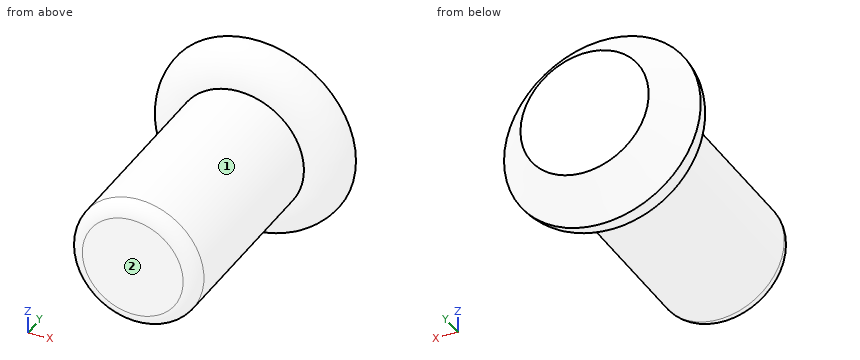
from build123d import *

# Parameters (mm, degrees)
F1_R     = 36.4721508719
F2_DEPTH = 25.399999693
F3_SIZE  = 12.7
F4_R     = 12.69999
F5_R     = 23.7721508719
F6_DEPTH = 101.6
F7_R     = 5.08


# Not quite as in the source:
# - a fillet or chamfer is up to 0.001 mm smaller than in the source, because OpenCascade refuses the exact size


with BuildPart() as f2:
    # F1 (on face) → F2 (new body)
    with BuildSketch(Plane.XZ):
        with Locations((27.7979820967, -14.2051279545)):
            Circle(F1_R)
    extrude(amount=-F2_DEPTH)

    # F3
    f3_edges = [f2.edges().sort_by_distance(p)[0] for p in [
        (-8.674169, 25.4, -14.205128),
    ]]
    chamfer(f3_edges, length=F3_SIZE)

    # F4 (radius 12.7 in the source; OpenCascade refuses exactly that, so slightly less here)
    f4_edges = [f2.edges().sort_by_distance(p)[0] for p in [
        (-8.674169, 0, -14.205128),
    ]]
    fillet(f4_edges, radius=F4_R)

    # F5 (on face) → F6 (join)
    with BuildSketch(Plane(origin=(0, 25.399999693, 0), x_dir=(-1, 0, 0), z_dir=(0, 1, 0))):
        with Locations((-27.7979820967, -14.2051279545)):
            Circle(F5_R)
    extrude(amount=-F6_DEPTH)

    # F7
    f7_edges = [f2.edges().sort_by_distance(p)[0] for p in [
        (51.570133, -76.2, -14.205128),
    ]]
    fillet(f7_edges, radius=F7_R)


solid = f2.part
CAD build for the part. Positions are in the model's coordinates, mm. Face numbers are marked on the shaded views. A direction names the side the tool comes from. Coordinates: 2 decimals unless noted, no trailing zeros. Order: outer loops, then holes, each group sorted by start corner. A loop starts at its lowest first (then second) coordinate and runs counter-clockwise, first axis right, second up.
Item 1: 3-axis set-ups, long thin cutter, end or side, ignore diameter. For the marked faces 1 and 2: which of +Z, -Z, +X, -X, +Y, -Y reach the whole face in a straight line?
Check sheet entries:
face 1: -Y
face 2: +Z, -Z, +X, -X, -Y
Item 2: Drill centre lines: L1, parallel to Z at x = 27.5, y = -44; L2, parallel to Y at x = 25, z = -45.5; L3, parallel to Y at x = 0, z = -12. Where is each one in solid material? Low to high.
Check sheet entries:
L1: z = -37.98 to 9.57
L2: y = 2.56 to 17.75
L3: y = 0.68 to 21.29
Item 3: Band-saw the part on A-A on y = 15. List the corners of the cut face in (x, z), plus the area to 3 significant figures.
Check sheet entries:
outline: circle Ø68.34 at (27.8, -14.21)
area: 3,670 mm2
Item 4: Pin check, flat tips, straight feed: pin 1 Ø4 at (x, z) = (-1, 1.5) entering from -Y; pin 2 Ø4 at (x, y) = (4, 9.5) entering from -Z; pin 3 Ø2 at (x, y) = (17.5, -64) entering from +Z. Stop position of each tip, or through.
Check sheet entries:
pin 1: stops at y = 2.12
pin 2: stops at z = -43.04
pin 3: stops at z = 7.67
Item 5: Band-saw the part on B-B on y = -58. List the corners of the cut face in (x, z).
Check sheet entries:
outline: circle Ø47.54 at (27.8, -14.21)
